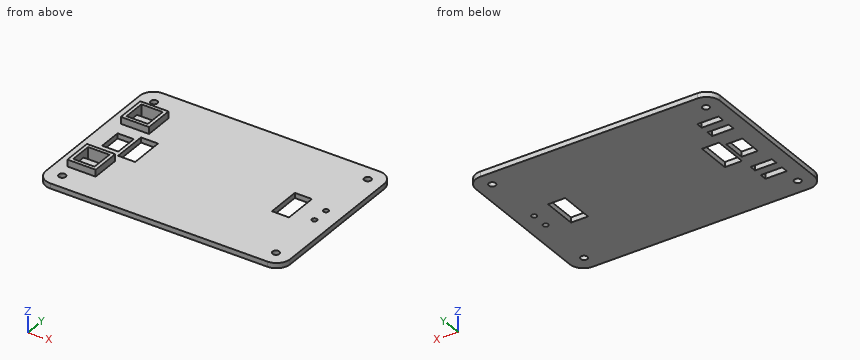
Autodesk Fusion 360 part; units mm, degrees
sketch "Boceto1" plane through (0, 0, 0) normal (0, 0, 1) x (1, 0, 0)
  line L0 (71.5, 0) -> (-71.5, 0)
  line L1 (0, -49) -> (0, 49)
  line L2 (-71.5, 49) -> (71.5, 49)
  line L3 (71.5, 49) -> (71.5, -49)
  line L4 (71.5, -49) -> (-71.5, -49)
  line L5 (-71.5, -49) -> (-71.5, 49)
  line L6 (-71.5, 49) -> (71.5, -49) construction
  line L7 (71.5, 49) -> (-71.5, -49) construction
  dimension "d1" = 143
  dimension "d2" = 98
extrude "Extruir1" add sketch "Boceto1" along normal blind 3
sketch "Boceto2" plane through (0, 0, 3) normal (0, 0, 1) x (-1, 0, 0)
  line L0 (71.5, 49) -> (-71.5, 49)
  line L1 (-71.5, 49) -> (-71.5, -49)
  line L2 (-71.5, -49) -> (71.5, -49)
  line L3 (71.5, -49) -> (71.5, 49)
  line L4 (71.5, -49) -> (62.5, -49)
  line L5 (62.5, -49) -> (62.5, -40)
  line L6 (71.5, 49) -> (62.5, 49)
  line L7 (62.5, 49) -> (62.5, 40)
  line L8 (-71.5, 49) -> (-71.5, 40)
  line L9 (-71.5, 40) -> (-62.5, 40)
  line L10 (-71.5, -49) -> (-62.5, -49)
  line L11 (-62.5, -49) -> (-62.5, -40)
  circle A0 centre (62.5, -40) radius 2
  circle A1 centre (62.5, 40) radius 2
  circle A2 centre (-62.5, -40) radius 2
  circle A3 centre (-62.5, 40) radius 2
  dimension "d7" = 9
  dimension "d8" = 9
  dimension "d9" = 9
  dimension "d10" = 9
  dimension "d11" = 9
  dimension "d12" = 9
  dimension "d13" = 9
  dimension "d14" = 9
  dimension "d15" = 4
  dimension "d16" = 4
  dimension "d17" = 4
  dimension "d18" = 4
extrude "Extruir2" cut sketch "Boceto2" against normal blind 3 contours A1 | A3 | A2 | A0
fillet "Empalme2" radius 8 4 edges at (-71.5, -49, 1.5) (-71.5, 49, 1.5) (71.5, -49, 1.5) (71.5, 49, 1.5)
sketch "Boceto3" plane through (0, 0, 3) normal (0, 0, 1) x (-1, 0, 0)
  circle A0 centre (62.5, 40) radius 2
  circle A1 centre (-62.5, -40) radius 2
  circle A2 centre (62.5, -40) radius 2
  circle A3 centre (-62.5, 40) radius 2
  arc A4 (-71.5, -41) -> (-63.5, -49) centre (-63.5, -41) ccw
  line L0 (-63.5, -49) -> (63.5, -49)
  arc A5 (63.5, -49) -> (71.5, -41) centre (63.5, -41) ccw
  line L1 (71.5, -41) -> (71.5, 41)
  arc A6 (71.5, 41) -> (63.5, 49) centre (63.5, 41) ccw
  line L2 (63.5, 49) -> (-63.5, 49)
  arc A7 (-63.5, 49) -> (-71.5, 41) centre (-63.5, 41) ccw
  line L3 (-71.5, 41) -> (-71.5, -41)
  line L4 (-40, 0) -> (40, 0)
  line L5 (40, 10) -> (40, -10)
  line L6 (-40, 10) -> (-40, -10)
  line L7 (40, -10) -> (50, -10)
  line L8 (50, -10) -> (50, 10)
  line L9 (50, 10) -> (40, 10)
  line L10 (40, 10) -> (40, -10)
  line L11 (-40, -10) -> (-50, -10)
  line L12 (-50, -10) -> (-50, 10)
  line L13 (-50, 10) -> (-40, 10)
  line L14 (-40, 10) -> (-40, -10)
  dimension "d23" = 80
  dimension "d24" = 20
  dimension "d25" = 20
  dimension "d26" = 10
  dimension "d27" = 20
  dimension "d28" = 10
  dimension "d29" = 20
extrude "Extruir3" cut sketch "Boceto3" against normal blind 3 contours L5 L7 L8 L9 L10 | L6 L11 L12 L13 L14
sketch "Boceto4" plane through (0, 0, 3) normal (0, 0, 1) x (-1, 0, 0)
  line L0 (50, -10) -> (40, -10)
  line L1 (40, -10) -> (40, 10)
  line L2 (40, 10) -> (50, 10)
  line L3 (50, 10) -> (50, -10)
  line L4 (-50, -10) -> (-50, 10)
  line L5 (-50, 10) -> (-40, 10)
  line L6 (-40, 10) -> (-40, -10)
  line L7 (-40, -10) -> (-50, -10)
  circle A0 centre (62.5, 40) radius 2
  circle A1 centre (-62.5, -40) radius 2
  circle A2 centre (62.5, -40) radius 2
  circle A3 centre (-62.5, 40) radius 2
  arc A4 (-71.5, -41) -> (-63.5, -49) centre (-63.5, -41) ccw
  line L8 (-63.5, -49) -> (63.5, -49)
  arc A5 (63.5, -49) -> (71.5, -41) centre (63.5, -41) ccw
  line L9 (71.5, -41) -> (71.5, 41)
  arc A6 (71.5, 41) -> (63.5, 49) centre (63.5, 41) ccw
  line L10 (63.5, 49) -> (-63.5, 49)
  arc A7 (-63.5, 49) -> (-71.5, 41) centre (-63.5, 41) ccw
  line L11 (-71.5, 41) -> (-71.5, -41)
  line L12 (71.5, 0) -> (61.5, 0)
  line L13 (61.5, 6.75) -> (61.5, -6.75)
  line L14 (61.5, -6.75) -> (52, -6.75)
  line L15 (61.5, 6.75) -> (52, 6.75)
  line L16 (52, 6.75) -> (52, -6.75)
  dimension "d32" = 10
  dimension "d33" = 13.5
  dimension "d34" = 9.5
  dimension "d35" = 9.5
extrude "Extruir4" cut sketch "Boceto4" against normal blind 3 contours L13 L14 L15 L16
sketch "Boceto5" plane through (0, 0, 3) normal (0, 0, 1) x (-1, 0, 0)
  line L0 (52, -6.75) -> (52, 6.75)
  line L1 (52, 6.75) -> (61.5, 6.75)
  line L2 (61.5, 6.75) -> (61.5, -6.75)
  line L3 (61.5, -6.75) -> (52, -6.75)
  line L4 (50, -10) -> (40, -10)
  line L5 (40, -10) -> (40, 10)
  line L6 (40, 10) -> (50, 10)
  line L7 (50, 10) -> (50, -10)
  line L8 (-50, -10) -> (-50, 10)
  line L9 (-50, 10) -> (-40, 10)
  line L10 (-40, 10) -> (-40, -10)
  line L11 (-40, -10) -> (-50, -10)
  circle A0 centre (62.5, 40) radius 2
  circle A1 centre (-62.5, -40) radius 2
  circle A2 centre (62.5, -40) radius 2
  circle A3 centre (-62.5, 40) radius 2
  arc A4 (-71.5, -41) -> (-63.5, -49) centre (-63.5, -41) ccw
  line L12 (-63.5, -49) -> (63.5, -49)
  arc A5 (63.5, -49) -> (71.5, -41) centre (63.5, -41) ccw
  line L13 (71.5, -41) -> (71.5, 41)
  arc A6 (71.5, 41) -> (63.5, 49) centre (63.5, 41) ccw
  line L14 (63.5, 49) -> (-63.5, 49)
  arc A7 (-63.5, 49) -> (-71.5, 41) centre (-63.5, 41) ccw
  line L15 (-71.5, 41) -> (-71.5, -41)
  line L16 (56.75, 6.75) -> (56.75, 16.75)
  line L17 (56.75, -6.75) -> (56.75, -16.75)
  line L18 (63, 16.75) -> (50.5, 16.75)
  line L19 (63, -16.75) -> (50.5, -16.75)
  line L20 (50.5, 16.75) -> (50.5, 29.75)
  line L21 (50.5, -16.75) -> (50.5, -29.75)
  line L22 (50.5, -29.75) -> (63, -29.75)
  line L23 (63, -29.75) -> (63, -16.75)
  line L24 (50.5, 29.75) -> (63, 29.75)
  line L25 (63, 29.75) -> (63, 16.75)
  line L26 (50.5, 25.6389) -> (50.5, 20.6389)
  line L27 (50.5, -20.8611) -> (50.5, -25.8611)
  line L28 (50.5, -25.8611) -> (63, -25.8611)
  line L29 (50.5, -20.8611) -> (63, -20.8611)
  line L30 (50.5, 20.6389) -> (63, 20.6389)
  line L31 (50.5, 25.6389) -> (63, 25.6389)
  line L32 (65, -31.75) -> (65, -14.75)
  line L33 (65, -14.75) -> (48.5, -14.75)
  line L34 (48.5, -14.75) -> (48.5, -31.75)
  line L35 (48.5, -31.75) -> (65, -31.75)
  line L36 (65, 31.75) -> (65, 14.75)
  line L37 (65, 14.75) -> (48.5, 14.75)
  line L38 (48.5, 14.75) -> (48.5, 31.75)
  line L39 (48.5, 31.75) -> (65, 31.75)
  point P0 (50.5, 23.1389)
  point P1 (50.5, -23.3611)
  dimension "d38" = 10
  dimension "d39" = 10
  dimension "d40" = 12.5
  dimension "d41" = 12.5
  dimension "d42" = 13
  dimension "d43" = 13
  dimension "d44" = 12.5
  dimension "d45" = 12.5
  dimension "d46" = 5
  dimension "d47" = 5
  dimension "d48" = 2
  dimension "d49" = -2
extrude "Extruir5" add sketch "Boceto5" along normal blind 4 contours L36 L37 L38 L39 | L32 L33 L34 L35
extrude "Extruir6" cut sketch "Boceto5" against normal blind 3 contours L18 L20 L25 L30 | L19 L21 L23 L29 | L21 L22 L23 L28 | L20 L24 L25 L31
sketch "Boceto6" plane through (0, 0, 3) normal (0, 0, 1) x (-1, 0, 0)
  line L0 (48.5, -31.75) -> (48.5, -14.75)
  line L1 (48.5, -14.75) -> (65, -14.75)
  line L2 (65, -14.75) -> (65, -31.75)
  line L3 (65, -31.75) -> (48.5, -31.75)
  line L4 (52, -6.75) -> (52, 6.75)
  line L5 (52, 6.75) -> (61.5, 6.75)
  line L6 (61.5, 6.75) -> (61.5, -6.75)
  line L7 (61.5, -6.75) -> (52, -6.75)
  line L8 (50, -10) -> (40, -10)
  line L9 (40, -10) -> (40, 10)
  line L10 (40, 10) -> (50, 10)
  line L11 (50, 10) -> (50, -10)
  line L12 (-50, -10) -> (-50, 10)
  line L13 (-50, 10) -> (-40, 10)
  line L14 (-40, 10) -> (-40, -10)
  line L15 (-40, -10) -> (-50, -10)
  circle A0 centre (62.5, 40) radius 2
  circle A1 centre (-62.5, -40) radius 2
  circle A2 centre (62.5, -40) radius 2
  circle A3 centre (-62.5, 40) radius 2
  arc A4 (-71.5, -41) -> (-63.5, -49) centre (-63.5, -41) ccw
  line L16 (-63.5, -49) -> (63.5, -49)
  arc A5 (63.5, -49) -> (71.5, -41) centre (63.5, -41) ccw
  line L17 (71.5, -41) -> (71.5, 41)
  arc A6 (71.5, 41) -> (63.5, 49) centre (63.5, 41) ccw
  line L18 (63.5, 49) -> (-63.5, 49)
  arc A7 (-63.5, 49) -> (-71.5, 41) centre (-63.5, 41) ccw
  line L19 (-71.5, 41) -> (-71.5, -41)
  line L20 (48.5, 31.75) -> (65, 31.75)
  line L21 (65, 31.75) -> (65, 14.75)
  line L22 (65, 14.75) -> (48.5, 14.75)
  line L23 (48.5, 14.75) -> (48.5, 31.75)
  line L24 (-71.5, 0) -> (-61.5, 0)
  line L25 (-61.5, -5) -> (-61.5, 5)
  circle A8 centre (-61.5, 5) radius 1.5
  circle A9 centre (-61.5, -5) radius 1.5
  dimension "d54" = 10
  dimension "d55" = 10
  dimension "d56" = 3
  dimension "d57" = 3
extrude "Extruir7" cut sketch "Boceto6" against normal blind 3 contours A8 | A9
Part model, mm, in its own coordinate system. Give positions to 0.01 mm unless a question says otherwise; leave off trailing zeros. Order: outer loops, then holes, each group sorted by start corner. A loop starts at its lowest first (then second) coordinate and runs counter-clockwise, first axis right, second up. Notation, with made-up numbers: M 26,-8.5 L 74,-8.5 A23 ccw 74,5.5 Z; hole C 80,70.25 d4. An arc over 180 degrees is marked long. Use a Markdown table: item, result. Add a question column.
(1) Saw through at A-A, the plane z = 5.5. Give the cut face in (x, y).
(2) Saw through at D-D, the plane x = -31.5. Give the cut face in (y, z).
(3) Probe line 1 along X through (y, z) = (-40, 2.35); line 2 along Y through (x, z) = (-64.5, 4.25); line 3 along Y through (x, z) = (-44, 2.5). List the from-to ranges inside material, lowest first. Write a range as [from, to].
(4) Saw through at B-B, the plane y = 5. Give the cut face in (x, z).
(5) Saw through at C-C, the plane x = -54. Give the number of separate pieces and of enclosed holes in the cut face, and give its area (4 significant figures).
(6) Drop flat-ended pins along their axis: P1, Ø5, axis at x = -8, y = -15.5, coming from the +Z side; P2, Ø3.5, axis at x = -54, z = 5, coming from the +Y side. Give the stop position or say it passes through.
Answer key:
| question | item | result |
|---|---|---|
| 1 | outline | M -65,-31.75 L -48.5,-31.75 L -48.5,-14.75 L -65,-14.75 Z; M -65,14.75 L -48.5,14.75 L -48.5,31.75 L -65,31.75 Z; hole M -63,-29.75 L -50.5,-29.75 L -50.5,-16.75 L -63,-16.75 Z; hole M -63,16.75 L -50.5,16.75 L -50.5,29.75 L -63,29.75 Z |
| 2 | outline | M -49,0 L 49,0 L 49,3 L -49,3 Z |
| 3 | line 1 | [-71.5, -64.5], [-60.5, 60.5], [64.5, 71.5] |
| 3 | line 2 | [-31.75, -14.75], [14.75, 31.75] |
| 3 | line 3 | [-49, -10], [10, 49] |
| 4 | outline | M -71.5,0 L -61.5,0 L -61.5,3 L -71.5,3 Z; M -52,0 L -50,0 L -50,3 L -52,3 Z; M -40,0 L 40,0 L 40,3 L -40,3 Z; M 50,0 L 60,0 L 60,3 L 50,3 Z; M 63,0 L 71.5,0 L 71.5,3 L 63,3 Z |
| 5 | separate pieces | 6 |
| 5 | enclosed holes | 0 |
| 5 | area | 237.5 mm^2 |
| 6 | P1 | z = 3 |
| 6 | P2 | y = 31.75 |
